```python
from build123d import *

# Parameters (mm, degrees)
SKETCH_1_W          = 50
SKETCH_1_H          = 50
EXTRUDE_1_DEPTH     = 10
SKETCH_2_W          = 30
SKETCH_2_H          = 10
EXTRUDE_2_DEPTH     = 30
SKETCH_3_R          = 10
CUT_EXTRUDE_1_DEPTH = 30


with BuildPart() as part:
    # 草图1 → 凸台-拉伸1 (new body)
    with BuildSketch(Plane.XY):
        Rectangle(SKETCH_1_W, SKETCH_1_H)
    extrude(amount=EXTRUDE_1_DEPTH)

    # 草图2 → 凸台-拉伸2 (add)
    with BuildSketch(Plane(origin=(0, 0, 0), x_dir=(-1, 0, 0), z_dir=(0, 0, -1))):
        Rectangle(SKETCH_2_W, SKETCH_2_H)
    extrude(amount=EXTRUDE_2_DEPTH)

    # 草图3 → 切除-拉伸1 (cut)
    with BuildSketch(Plane(origin=(0, 5, 0), x_dir=(1, 0, 0), z_dir=(0, 1, 0))):
        with Locations(Location((0, 15.717133963, 0), (0, 0, 180))):
            Circle(SKETCH_3_R)
    extrude(amount=-CUT_EXTRUDE_1_DEPTH, mode=Mode.SUBTRACT)


solid = part.part
```
Can you work these out from the model? Positions are in its coordinate system, mm. A direction names the side the tool comes from. Give positions to 0.01 mm unless a question says otherwise; leave off trailing zeros. Write each loop counter-clockwise with the first axis right and the second up, starting at its lowest first coordinate (ties: lowest second). Pieces come first, ordered by that corner, then holes. Notation, with made-up numbers: (31.5, -13) - (80.5, -13) arc R25 ccw to (80.5, 15) - close; hole circle Ø4 at (-13, 66). An arc over 180 degrees is marked (long way). Write item = value, one per line. Start each with the question number.
1. Please list where these lines run through material, in increasing order: line 1 (Z direction, x = 0, y = 2); line 2 (Y direction, x = -12.5, z = -27); line 3 (Z direction, x = -7, y = -12.5).
2. Thinking about a two-plate mould opening in Z: for faces 5 (the face through (0, 0, -30)), 6 (the face through (2.17, 0.07, -25.48)), 7 (the face through (15, 0, -15)), 8 (the face through (0, 0, 10)), which applies, released by +Z, released by -Z, zero draft, split by the parting line, or undercut?
3. On a 3-axis mill with a long thin cutter (end or side, diameter ignored), from which of +Z, -Z, +X, -X, +Y, -Y can I reach the whole of each face in a straight line? I mean faces 1 (the face through (7, -5, -8)), 2 (the face through (-15, 0, -15)), 3 (the face through (0, 25, 5)), 4 (the face through (7, 5, -8)). Say none if no direction works.
4. Imagine slicing it at D-D (y = -10). Please give me the cut outline in (x, z), and give its area (3 significant figures).
5. For pin 1 (10 mm diameter, centred on x = 14, y = 11.5, fed in from -Z); pin 2 (10 mm diameter, centred on x = 12.5, z = -17, fed in from +Y); pin 3 (5 mm diameter, centred on y = 0.5, z = -21, fed in from -X), each with a flat end and sliding along its axis, tell me the tip position at first contact or that it passes through.
6. Imagine slicing it at C-C (z = -9). Please give me the cut outline in (x, y).
7. Imagine slicing it at B-B (x = -13.5). Please give me the cut outline in (y, z).
8. Imagine slicing it at A-A (x = 0). Please give me the cut outline in (y, z).
Worked answers:
q1.line_1 = -30 to -25.72, -5.72 to 10
q1.line_2 = -5 to 5
q1.line_3 = 0 to 10
q2.face_5 = released by -Z
q2.face_6 = undercut
q2.face_7 = zero draft
q2.face_8 = released by +Z
q3.face_1 = -Z, +X, -X, -Y
q3.face_2 = -Z, -X, +Y, -Y
q3.face_3 = +Z, -Z, +X, -X, +Y
q3.face_4 = -Z, +X, -X, +Y
q4.outline = (-25, 0) - (25, 0) - (25, 10) - (-25, 10) - close
q4.area = 500 mm2
q5.pin_1 = 0
q5.pin_2 = 5
q5.pin_3 = -15
q6.outline = (-15, -5) - (-7.41, -5) - (-7.41, 5) - (-15, 5) - close; (7.41, -5) - (15, -5) - (15, 5) - (7.41, 5) - close
q7.outline = (-25, 0) - (-5, 0) - (-5, -30) - (5, -30) - (5, 0) - (25, 0) - (25, 10) - (-25, 10) - close
q8.outline = (-25, 0) - (-5, 0) - (-5, -5.72) - (5, -5.72) - (5, 0) - (25, 0) - (25, 10) - (-25, 10) - close; (-5, -30) - (5, -30) - (5, -25.72) - (-5, -25.72) - close
